from build123d import *

# Parameters (mm, degrees)
BOSS_EXTRUDE1_DEPTH = 4
SKETCH3_R           = 2
CUT_EXTRUDE1_DEPTH  = 10
CUT_EXTRUDE2_DEPTH  = 167.695623666


with BuildPart() as part:
    # Sketch1 → Boss-Extrude1 (new body)
    with BuildSketch(Plane.XY):
        with BuildLine():
            Line((65.293896859, 140.79456376), (-65.293896859, 140.79456376))
            ThreePointArc((-65.293896859, 140.79456376), (-83.510437362, 132.343917874), (-88.822955159, 112.978151212))
            ThreePointArc((-88.822955159, 112.978151212), (-82.121571276, 106.62300147), (-74.161000128, 111.305498795))
            Line((-74.161000128, 111.305498795), (-70.965431907, 118.996456291))
            ThreePointArc((-70.965431907, 118.996456291), (-68.695430494, 121.757834263), (-65.274420897, 122.79456376))
            Line((-65.274420897, 122.79456376), (65.274420897, 122.79456376))
            ThreePointArc((65.274420897, 122.79456376), (68.695430494, 121.757834263), (70.965431907, 118.996456291))
            Line((70.965431907, 118.996456291), (74.161000128, 111.305498795))
            ThreePointArc((74.161000128, 111.305498795), (82.121571276, 106.62300147), (88.822955159, 112.978151212))
            ThreePointArc((88.822955159, 112.978151212), (83.510437362, 132.343917874), (65.293896859, 140.79456376))
        make_face()
    extrude(amount=BOSS_EXTRUDE1_DEPTH)

    # Sketch3 → Cut-Extrude1 (cut)
    with BuildSketch(Plane.XY.offset(4)):
        with Locations((-47.324700565, 132.53476761)):
            Circle(SKETCH3_R)
        with Locations((47.324700565, 132.53476761)):
            Circle(SKETCH3_R)
    extrude(amount=-CUT_EXTRUDE1_DEPTH, mode=Mode.SUBTRACT)

    # Sketch4 → Cut-Extrude2 (cut, through all)
    with BuildSketch(Plane.XY.offset(4)):
        Polygon((-11.999700565, 135.79456376), (-11.999700565, 126.79456376), (-11.999700565, 122.79456376), (19.000299435, 122.79456376), (19.000299435, 126.79456376), (19.000299435, 135.79456376), align=None)
    extrude(amount=-CUT_EXTRUDE2_DEPTH, mode=Mode.SUBTRACT)


solid = part.part
Input: part model. Units: mm. Frame: model coordinates. A direction names the side the tool comes from. Coordinates: 2 decimals unless noted, no trailing zeros. Loops run counter-clockwise (first coordinate to the right, second up) from the corner with the lowest first, then second, coordinate; pieces in that order, holes last.
Q1. Cut plane C-C (x = -19). Output: boundary loops of the cut face in (y, z), then the cut area to 3 significant figures.
Q2. Material intervals for line 1 (X direction, y = 132.5, z = 1.55) (3 decimals); line 2 (Y direction, x = 50.5, z = 1); line 3 (X direction, y = 110, z = 0.9), sorted ascending.
Q3. Contact query for flat-ended pins moving along their axis: pin 1 (1.5 mm diameter, centred on x = -7.5, z = 1, fed in from -Y); pin 2 (2 mm diameter, centred on x = -16.5, z = 0.5, fed in from -Y); pin 3 (2 mm diameter, centred on y = 131, z = 1, fed in from +X). Output: stop coordinate, or through.
Q4. Cut plane D-D (x = 69). Output: boundary loops of the cut face in (y, z).
Q5. Cut plane A-A (y = 117.5). Output: boundary loops of the cut face in (x, z), then the cut area to 3 significant figures.
Q6. Cut plane B-B (z = 1.55). Output: boundary loops of the cut face in (x, y).
Q7. Set-up query: faces 5 (the face through (-1, 139, 0)), 6 (the face through (19, 129, 2)). Return all of +Z, -Z, +X, -X, +Y, -Y with unobstructed straight access to the full face (end or side cutting, diameter ignored); none if empty.
Q8. Draft query along Y for faces 1 (the face through (-1, 139, 4)), 2 (the face through (-46.4, 130.76, 2.03)), 3 (the face through (48.25, 130.76, 2.03)), 4 (the face through (1, 140.795, 2)). Return one class per face: +Y half, -Y half, draft (parallel to the pull), parting line (faces both ways), or undercut.
Working result:
1. outline: (122.79, 0) - (140.79, 0) - (140.79, 4) - (122.79, 4) - close
1. area: 72.0 mm2
2. line 1: x = -83.377 to -49.324, -45.325 to -12, 19 to 45.325, 49.324 to 83.377
2. line 2: y = 122.79 to 140.79
2. line 3: x = -87.64 to -74.86, 74.86 to 87.64
3. pin 1: stops at y = 135.79
3. pin 2: stops at y = 122.79
3. pin 3: stops at x = 85.26
4. outline: (121.54, 0) - (140.5, 0) - (140.5, 4) - (121.54, 4) - close
5. outline: (-89.15, 0) - (-71.59, 0) - (-71.59, 4) - (-89.15, 4) - close; (71.59, 0) - (89.15, 0) - (89.15, 4) - (71.59, 4) - close
5. area: 140 mm2
6. outline: (-88.82, 112.98) arc R7.68 ccw to (-74.16, 111.31) - (-70.97, 119) arc R6.16 cw to (-65.27, 122.79) - (-12, 122.79) - (-12, 135.79) - (19, 135.79) - (19, 122.79) - (65.27, 122.79) arc R6.16 cw to (70.97, 119) - (74.16, 111.31) arc R7.68 ccw to (88.82, 112.98) arc R23.86 ccw to (65.29, 140.79) - (-65.29, 140.79) arc R23.86 ccw to start; hole circle Ø4 at (-47.32, 132.53); hole circle Ø4 at (47.32, 132.53)
7. face 5: -Z, +X, -X, +Y, -Y
7. face 6: +Z, -Z, -Y
8. face 1: draft
8. face 2: undercut
8. face 3: undercut
8. face 4: +Y half
